```python
from build123d import *

# Parameters (mm, degrees)
SKETCH1_W           = 7.8
SKETCH1_H           = 3.2
BOSS_EXTRUDE1_DEPTH = 7.8
SKETCH2_R           = 2.4
BOSS_EXTRUDE2_DEPTH = 1.6
SHELL1_T            = -0.7
SKETCH3_W           = 2.8
SKETCH3_H           = 3.2
BOSS_EXTRUDE3_DEPTH = 1.5
BOSS_EXTRUDE4_DEPTH = 3.2
FILLET1_R           = 0.75
FILLET2_R           = 0.75
SKETCH6_R           = 0.424931422
CUT_EXTRUDE1_DEPTH  = 1.6


with BuildPart() as part:
    # Sketch1 → Boss-Extrude1 (new body)
    with BuildSketch(Plane.XY):
        with Locations((3.9, 1.6)):
            Rectangle(SKETCH1_W, SKETCH1_H)
    extrude(amount=-BOSS_EXTRUDE1_DEPTH)

    # Sketch2 → Boss-Extrude2 (add)
    with BuildSketch(Plane(origin=(0, 3.2, 0), x_dir=(1, 0, 0), z_dir=(0, 1, 0))):
        with Locations(Location((3.9, 3.9, 0), (0, 0, 270))):
            Circle(SKETCH2_R)
    extrude(amount=BOSS_EXTRUDE2_DEPTH)

    # Shell1
    shell1_openings = [part.faces().sort_by_distance(p)[0] for p in [
        (3.9, 0, -3.9),
    ]]
    offset(amount=SHELL1_T, openings=shell1_openings, kind=Kind.INTERSECTION)

    # Sketch3 → Boss-Extrude3 (add)
    with BuildSketch(Plane.XY):
        with Locations((3.9, 1.6)):
            Rectangle(SKETCH3_W, SKETCH3_H)
    extrude(amount=BOSS_EXTRUDE3_DEPTH)

    # Sketch5 → Boss-Extrude4 (add)
    with BuildSketch(Plane(origin=(0, 3.2, 0), x_dir=(1, 0, 0), z_dir=(0, 1, 0))):
        with BuildLine():
            Line((0.960612309, -5.988310559), (2.416065979, -5.988310559))
            Line((2.416065979, -5.988310559), (2.416065979, -4.707262204))
            ThreePointArc((2.416065979, -4.707262204), (3.9, -2.988310559), (5.383934021, -4.707262204))
            Line((5.383934021, -4.707262204), (5.383934021, -5.988310559))
            Line((5.383934021, -5.988310559), (6.839387691, -5.988310559))
            ThreePointArc((6.839387691, -5.988310559), (3.9, -1.188310559), (0.960612309, -5.988310559))
        make_face()
    extrude(amount=-BOSS_EXTRUDE4_DEPTH)

    # Fillet1
    fillet1_edges = [part.edges().sort_by_distance(p)[0] for p in [
        (2.5, 1.6, 0),
        (2.5, 1.6, 1.5),
    ]]
    fillet(fillet1_edges, radius=FILLET1_R)

    # Fillet2
    fillet2_edges = [part.edges().sort_by_distance(p)[0] for p in [
        (5.3, 1.6, 0),
        (5.3, 1.6, 1.5),
    ]]
    fillet(fillet2_edges, radius=FILLET2_R)

    # Sketch6 → Cut-Extrude1 (cut)
    with BuildSketch(Plane.XZ):
        with Locations(Location((3.7900748, 0.342701654, 0), (0, 0, 270))):
            Circle(SKETCH6_R)
    extrude(amount=-CUT_EXTRUDE1_DEPTH, mode=Mode.SUBTRACT)


solid = part.part
```
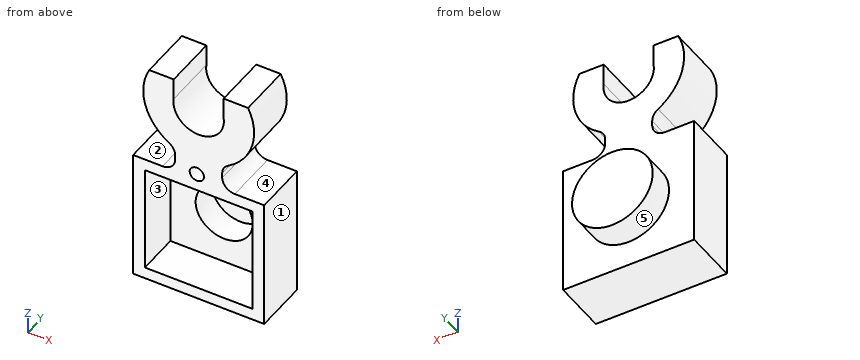
Can you work these out from the model? Positions are in its coordinate system, mm. Face numbers are marked on the shaded views. A direction names the side the tool comes from. Round coordinates to 2 decimals unless told otherwise and drop trailing zeros. Loops run counter-clockwise (first coordinate to the right, second up) from the corner with the lowest first, then second, coordinate; pieces in that order, holes last. Notation, with made-up numbers: M 84.5,-26.75 L 123.5,-26.75 A20 cw 123.5,-4.75 Z; hole C 10.25,-32 d1. An arc over 180 degrees is marked long. Answer in a Markdown table with one row per item.
1. If we section it at D-D, the plane z = 4.25: Please give me the cut outline in (x, y).
Established:
| item | result |
|---|---|
| outline | M 0.61,0 L 2.42,0 L 2.42,3.2 L 0.61,3.2 Z; M 5.38,0 L 7.19,0 L 7.19,3.2 L 5.38,3.2 Z |
2. If we section it at A-A, the plane y = 1.75: Please give me the cut outline in (x, z), plus the area to 3 significant figures.
Established:
| item | result |
|---|---|
| outline | M 0,-7.8 L 7.8,-7.8 L 7.8,0 L 6.05,0 A0.75 cw 5.3,0.75 L 5.3,1.06 A0.75 cw 5.65,1.69 A3.3 ccw 6.84,5.99 L 5.38,5.99 L 5.38,4.71 A1.5 cw long 2.42,4.71 L 2.42,5.99 L 0.96,5.99 A3.3 ccw 2.15,1.69 A0.75 cw 2.5,1.06 L 2.5,0.75 A0.75 cw 1.75,0 L 0,0 Z; hole M 0.7,-7.1 L 7.1,-7.1 L 7.1,-0.7 L 0.7,-0.7 Z |
| area | 42.5 mm² |
3. Please list where these lines run through material, in increasing order: line 1 (X direction, y = 1.4, z = -4.25); line 2 (X direction, y = 3.25, z = -3.9); line 3 (Z direction, x = 1, y = 0.55). Write a range as from..to.
Established:
| item | result |
|---|---|
| line 1 | 0..0.7, 7.1..7.8 |
| line 2 | 1.5..2.2, 5.6..6.3 |
| line 3 | -7.8..-7.1, -0.7..0, 2.91..5.99 |
4. If we section it at B-B, the plane x = 2: Please give me the cut outline in (y, z).
Established:
| item | result |
|---|---|
| outline | M 0,-7.8 L 3.2,-7.8 L 3.2,-5.37 L 4.8,-5.37 L 4.8,-2.43 L 3.2,-2.43 L 3.2,0.04 L 0,0.04 L 0,-0.7 L 2.5,-0.7 L 2.5,-7.1 L 0,-7.1 Z; M 0,1.79 L 3.2,1.79 L 3.2,5.99 L 0,5.99 Z |
5. On a 3-axis mill with a long thin cutter (end or side, diameter ignored), from which of +Z, -Z, +X, -X, +Y, -Y can I reach the whole of each face in a straight line? I mean the marked faces 1, 2, 3, 4 and 5. Say none if no direction works.
Established:
| item | result |
|---|---|
| face 1 | +Z, -Z, +X, +Y, -Y |
| face 2 | -X, +Y, -Y |
| face 3 | -Y |
| face 4 | +X, +Y, -Y |
| face 5 | +Y |
6. I'm going to push flat-ended pins straight in: pin 1 Ø2 at (x, z) = (3.9, -3.9) entering from -Y; pin 2 Ø1 at (x, y) = (3.5, 3) entering from +Z; pin 3 Ø1.7 at (x, z) = (3, -3) entering from -Y. Where does each tip first touch, or does it pass through?
Established:
| item | result |
|---|---|
| pin 1 | y = 4.1 |
| pin 2 | z = 3.29 |
| pin 3 | y = 2.5 |
7. If we section it at C-C, the plane z = -3.9: Please give me the cut outline in (x, y).
Established:
| item | result |
|---|---|
| outline | M 0,0 L 0.7,0 L 0.7,2.5 L 2.2,2.5 L 2.2,4.1 L 5.6,4.1 L 5.6,2.5 L 7.1,2.5 L 7.1,0 L 7.8,0 L 7.8,3.2 L 6.3,3.2 L 6.3,4.8 L 1.5,4.8 L 1.5,3.2 L 0,3.2 Z |
